from build123d import *

# Parameters (mm, degrees)
SKETCH1_R               = 2.159
SKETCH1_R_2             = 28.5115
BOSS_EXTRUDE1_DEPTH     = 9.7155
SKETCH1_4_R             = 28.5115
SKETCH1_4_R_2           = 23.8125
FLUSH_BEZEL_DEPTH       = 9.7155
SKETCH1_5_R             = 28.5115
SKETCH1_5_R_2           = 23.8125
BOSS_EXTRUDE4_DEPTH     = 6.35
SKETCH2_R               = 25.3365
CUT_EXTRUDE1_DEPTH      = 7.35
CUT_EXTRUDE1_DEPTH_BACK = 9.7155
SKETCH3_R               = 28.5115
CUT_EXTRUDE2_DEPTH      = 7.35
SKETCH4_R               = 25.3365
SKETCH4_R_2             = 23.8125
BOSS_EXTRUDE7_DEPTH     = 1.5875


with BuildPart() as part:
    # Sketch1 → Boss-Extrude1 (new body)
    with BuildSketch(Plane.XY):
        with BuildLine():
            ThreePointArc((-24.49722379, -28.024879905), (-26.788104009, -26.788104009), (-28.024879905, -24.49722379))
            Line((-28.024879905, -24.49722379), (-30.1625, -14.199031657))
            Line((-30.1625, -14.199031657), (-30.1625, 14.199031657))
            Line((-30.1625, 14.199031657), (-28.024879905, 24.49722379))
            ThreePointArc((-28.024879905, 24.49722379), (-26.788104009, 26.788104009), (-24.49722379, 28.024879905))
            Line((-24.49722379, 28.024879905), (-14.199031657, 30.1625))
            Line((-14.199031657, 30.1625), (14.199031657, 30.1625))
            Line((14.199031657, 30.1625), (24.441349319, 28.268787691))
            ThreePointArc((24.441349319, 28.268787691), (26.949748619, 26.949748619), (28.268787691, 24.441349319))
            Line((28.268787691, 24.441349319), (30.1625, 14.199031657))
            Line((30.1625, 14.199031657), (30.1625, -14.199031657))
            Line((30.1625, -14.199031657), (28.024879905, -24.49722379))
            ThreePointArc((28.024879905, -24.49722379), (26.788104009, -26.788104009), (24.49722379, -28.024879905))
            Line((24.49722379, -28.024879905), (14.199031657, -30.1625))
            Line((14.199031657, -30.1625), (-14.199031657, -30.1625))
            Line((-14.199031657, -30.1625), (-24.49722379, -28.024879905))
        make_face()
        with Locations((-23.573172318, -23.573172318)):
            Circle(SKETCH1_R, mode=Mode.SUBTRACT)
        with Locations((23.573172318, -23.573172318)):
            Circle(SKETCH1_R, mode=Mode.SUBTRACT)
        with Locations((23.573172318, 23.573172318)):
            Circle(SKETCH1_R, mode=Mode.SUBTRACT)
        with Locations((-23.573172318, 23.573172318)):
            Circle(SKETCH1_R, mode=Mode.SUBTRACT)
        Circle(SKETCH1_R_2, mode=Mode.SUBTRACT)
        with BuildLine():
            Line((28.268787691, 24.441349319), (30.1625, 14.199031657))
            Line((30.1625, 14.199031657), (30.1625, 25.3873))
            ThreePointArc((30.1625, 25.3873), (28.763876302, 28.763876302), (25.3873, 30.1625))
            Line((25.3873, 30.1625), (14.199031657, 30.1625))
            Line((14.199031657, 30.1625), (24.441349319, 28.268787691))
            ThreePointArc((24.441349319, 28.268787691), (26.949748619, 26.949748619), (28.268787691, 24.441349319))
        make_face()
        with BuildLine():
            Line((-30.1625, 25.3873), (-30.1625, 14.199031657))
            Line((-30.1625, 14.199031657), (-28.024879905, 24.49722379))
            ThreePointArc((-28.024879905, 24.49722379), (-26.788104009, 26.788104009), (-24.49722379, 28.024879905))
            Line((-24.49722379, 28.024879905), (-14.199031657, 30.1625))
            Line((-14.199031657, 30.1625), (-25.3873, 30.1625))
            ThreePointArc((-25.3873, 30.1625), (-28.763876302, 28.763876302), (-30.1625, 25.3873))
        make_face()
        with BuildLine():
            Line((-25.3873, -30.1625), (-14.199031657, -30.1625))
            Line((-14.199031657, -30.1625), (-24.49722379, -28.024879905))
            ThreePointArc((-24.49722379, -28.024879905), (-26.788104009, -26.788104009), (-28.024879905, -24.49722379))
            Line((-28.024879905, -24.49722379), (-30.1625, -14.199031657))
            Line((-30.1625, -14.199031657), (-30.1625, -25.3873))
            ThreePointArc((-30.1625, -25.3873), (-28.763876302, -28.763876302), (-25.3873, -30.1625))
        make_face()
        with BuildLine():
            Line((24.49722379, -28.024879905), (14.199031657, -30.1625))
            Line((14.199031657, -30.1625), (25.3873, -30.1625))
            ThreePointArc((25.3873, -30.1625), (28.763876302, -28.763876302), (30.1625, -25.3873))
            Line((30.1625, -25.3873), (30.1625, -14.199031657))
            Line((30.1625, -14.199031657), (28.024879905, -24.49722379))
            ThreePointArc((28.024879905, -24.49722379), (26.788104009, -26.788104009), (24.49722379, -28.024879905))
        make_face()
    extrude(amount=BOSS_EXTRUDE1_DEPTH)

    # Sketch1_4 → Flush Bezel (add)
    with BuildSketch(Plane.XY):
        Circle(SKETCH1_4_R)
        Circle(SKETCH1_4_R_2, mode=Mode.SUBTRACT)
    extrude(amount=FLUSH_BEZEL_DEPTH)

    # Sketch1_5 → Boss-Extrude4 (add)
    with BuildSketch(Plane.XY):
        Circle(SKETCH1_5_R)
        Circle(SKETCH1_5_R_2, mode=Mode.SUBTRACT)
    extrude(amount=-BOSS_EXTRUDE4_DEPTH)

    # Sketch2 → Cut-Extrude1 (cut, two sides)
    with BuildSketch(Plane(origin=(0, 0, 0), x_dir=(-1, 0, 0), z_dir=(0, 0, -1))) as cut_extrude1_sk:
        Circle(SKETCH2_R)
    extrude(amount=CUT_EXTRUDE1_DEPTH, mode=Mode.SUBTRACT)
    extrude(cut_extrude1_sk.sketch, amount=-CUT_EXTRUDE1_DEPTH_BACK, mode=Mode.SUBTRACT)

    # Sketch3 → Cut-Extrude2 (cut, through all)
    with BuildSketch(Plane(origin=(0, 0, 0), x_dir=(-1, 0, 0), z_dir=(0, 0, -1))):
        Circle(SKETCH3_R)
    extrude(amount=CUT_EXTRUDE2_DEPTH, mode=Mode.SUBTRACT)

    # Sketch4 → Boss-Extrude7 (add)
    with BuildSketch(Plane.XY.offset(9.7155)):
        Circle(SKETCH4_R)
        Circle(SKETCH4_R_2, mode=Mode.SUBTRACT)
    extrude(amount=-BOSS_EXTRUDE7_DEPTH)


solid = part.part
Model file for the job. Use its own axes, mm. A direction names the side the tool comes from. Coordinates: 2 decimals unless noted, no trailing zeros. Write each loop counter-clockwise with the first axis right and the second up, starting at its lowest first coordinate (ties: lowest second). Pieces come first, ordered by that corner, then holes. Notation, with made-up numbers: (-30, -40) -> (-16, -40) arc R10 cw to (-16, -34) -> close; hole circle Ø1 at (-14, 5). An arc over 180 degrees is marked (long way). One line per item, written item: value. Start each with the question number.
1) Probe probe 1 along X at (y, z) = (24.5, 9); probe 2 along Y at (x, z) = (-22.5, 2); probe 3 along X at (y, z) = (-22, 5.5). List the from-to ranges inside material, lowest first.
2) Which spindle directions (+Z, -Z, +X, -X, +Y, -Y) get a long thin tool onto all of the face, cutting with end or side? Do faces 1 (the face through (-23, -7, 8.128)), 2 (the face through (25.568, -24.4, 4.79)). Say none if no direction does.
3) Slice it at C-C on z = 1. Write the cut outline in (x, y), then the cut area to 3 significant figures.
4) Pull direction Y, two halves, no side cores. Call faces 3 (the face through (-13.621, 21.364, 4.121)), 4 (the face through (0, 30.162, 5)), 5 (the face through (-28.8, -28.73, 4.79)): +Y half, -Y half, draft (parallel to the pull), parting line (faces both ways), or undercut.
5) Flat gauge pins, fed straight in: pin 1 Ø12 at (x, y) = (10, -21.5) entering from -Z; pin 2 Ø4 at (x, y) = (22.5, -5) entering from -Z. Where does each tip first touch, or does it go through?
6) Slice it at A-A on x = 0. Write the cut outline in (y, z), then the cut area to 3 significant figures.
Answers follow:
1. probe 1: -30.16 to -25.52, -21.62 to 21.62, 25.52 to 30.16
1. probe 2: -30.16 to -25.45, -21.7 to -11.65, 11.65 to 21.7, 25.45 to 30.16
1. probe 3: -30.16 to -25.05, -22.09 to -12.57, 12.57 to 22.09, 25.05 to 30.16
2. face 1: -Z
2. face 2: +Z, -Z
3. outline: (-30.16, -25.39) arc R4.78 ccw to (-25.39, -30.16) -> (25.39, -30.16) arc R4.78 ccw to (30.16, -25.39) -> (30.16, 25.39) arc R4.78 ccw to (25.39, 30.16) -> (-25.39, 30.16) arc R4.78 ccw to (-30.16, 25.39) -> close; hole circle Ø4.32 at (-23.57, -23.57); hole circle Ø4.32 at (-23.57, 23.57); hole circle Ø50.67 at (0, 0); hole circle Ø4.32 at (23.57, -23.57); hole circle Ø4.32 at (23.57, 23.57)
3. area: 1,540 mm2
4. face 3: undercut
4. face 4: +Y half
4. face 5: -Y half
5. pin 1: z = 0
5. pin 2: z = 8.13
6. outline: (-30.16, 0) -> (-25.34, 0) -> (-25.34, 8.13) -> (-23.81, 8.13) -> (-23.81, 9.72) -> (-30.16, 9.72) -> close; (23.81, 8.13) -> (25.34, 8.13) -> (25.34, 0) -> (30.16, 0) -> (30.16, 9.72) -> (23.81, 9.72) -> close
6. area: 98.6 mm2
